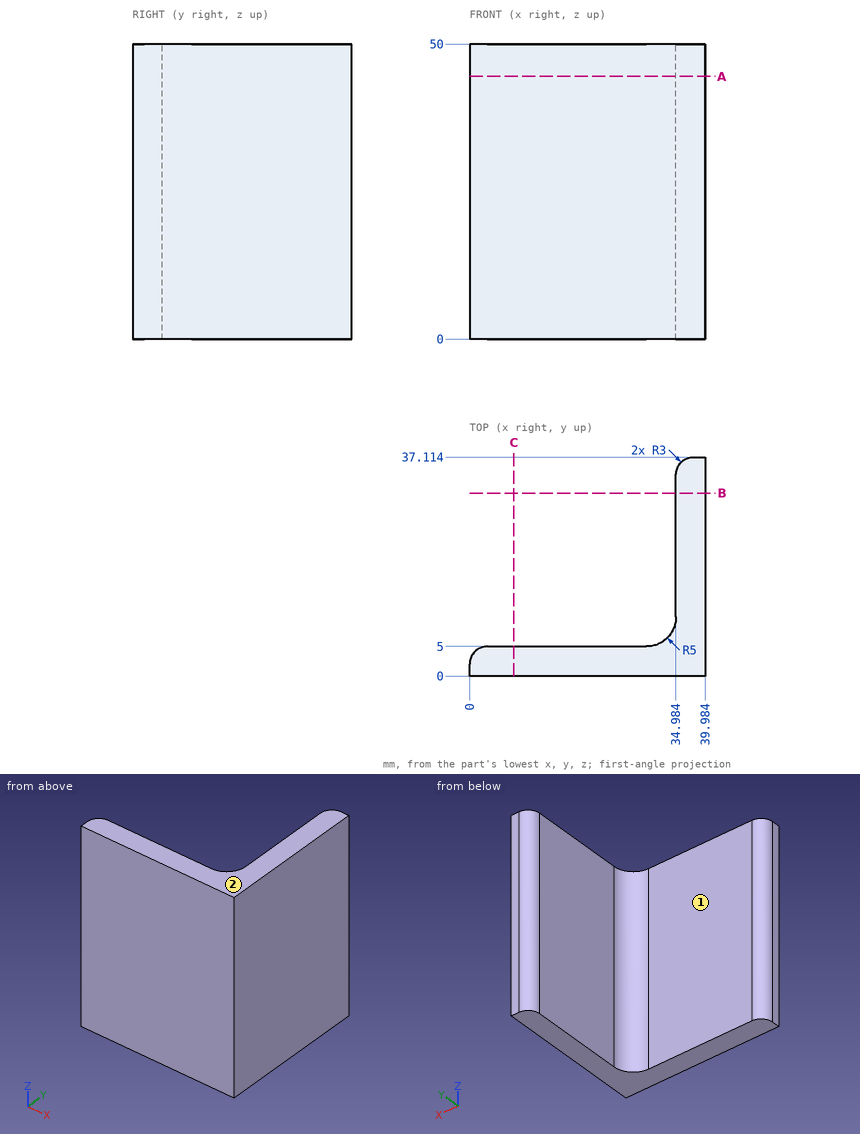
Geometry: see drawing. Coordinates: mm, zero at the bounding-box minimum. A direction names the side the tool comes from. Give positions to 0.01 mm unless a question says otherwise; leave off trailing zeros. Order: outer loops, then holes, each group sorted by start corner. A loop starts at its lowest first (then second) coordinate and runs counter-clockwise, first axis right, second up. Notation, with made-up numbers: (-26.5, 86) - (27.5, 86) arc R27 cw to (27.5, 118) - close; hole circle Ø1 at (16.25, 30.5). An arc over 180 degrees is marked (long way). One line per item, written item: value.
1. Line query: probe 1 along Y at (x, z) = (29.5, 18); probe 2 along X at (y, z) = (34, 22); probe 3 along Y at (x, z) = (37, 4). Output: solid intervals per line, ascending.
Determined:
probe 1: 0 to 5
probe 2: 34.98 to 39.98
probe 3: 0 to 36.95
2. Cut plane C-C, the plane x = 7.5. Output: boundary loops of the cut face in (y, z).
Determined:
outline: (0, 0) - (5, 0) - (5, 50) - (0, 50) - close
3. Pin query (flat end, axial travel): pin 1 Ø2 at (x, z) = (19.5, 43) entering from +Y; pin 2 Ø4 at (y, z) = (25, 34.5) entering from -X. Return the tip coordinate at first contact, or that it passes through.
Determined:
pin 1: y = 5
pin 2: x = 34.98
4. Cut plane A-A, the plane z = 44.5. Output: boundary loops of the cut face in (x, y), and give its area (3 significant figures).
Determined:
outline: (0, 0) - (39.98, 0) - (39.98, 37.11) - (37.98, 37.11) arc R3 ccw to (34.98, 34.11) - (34.98, 10) arc R5 cw to (29.98, 5) - (3, 5) arc R3 ccw to (0, 2) - close
area: 362 mm2
5. Reachability of the marked faces 1 and 2 from +Z, -Z, +X, -X, +Y, -Y: full face, straight path, thin tool, end or side. Return the list, or none.
Determined:
face 1: +Z, -Z, -X, +Y
face 2: +Z, +X, -X, +Y, -Y
6. Cut plane B-B, the plane y = 31. Output: boundary loops of the cut face in (x, z), and give its area (3 significant figures).
Determined:
outline: (34.98, 0) - (39.98, 0) - (39.98, 50) - (34.98, 50) - close
area: 250 mm2
